```python
from build123d import *

# Parameters (mm, degrees)
SKETCH1_W           = 18.8
SKETCH1_H           = 14.8
BOSS_EXTRUDE1_DEPTH = 5.2
SKETCH2_W           = 1.2
SKETCH2_H           = 0.8
CUT_EXTRUDE1_DEPTH  = 19.287700785
SKETCH3_W           = 1.2
SKETCH3_H           = 0.8
CUT_EXTRUDE2_DEPTH  = 19.287700785
SKETCH4_W           = 1.2
SKETCH4_H           = 0.8
CUT_EXTRUDE3_DEPTH  = 19.287700785
SKETCH5_W           = 1.2
SKETCH5_H           = 0.8
CUT_EXTRUDE4_DEPTH  = 19.287700785
SKETCH6_W           = 1.2
SKETCH6_H           = 0.8
CUT_EXTRUDE5_DEPTH  = 19.287700785
SKETCH7_W           = 1.2
SKETCH7_H           = 0.8
CUT_EXTRUDE6_DEPTH  = 19.287700785
SKETCH8_W           = 1.2
SKETCH8_H           = 0.8
CUT_EXTRUDE7_DEPTH  = 19.287700785
SKETCH9_W           = 1.2
SKETCH9_H           = 0.8
CUT_EXTRUDE8_DEPTH  = 19.287700785
SKETCH10_W          = 1.2
SKETCH10_H          = 0.8
CUT_EXTRUDE9_DEPTH  = 19.287700785
RIB1_REACH          = 15.045
SKETCH11_WALL_W     = 29.289078174
SKETCH11_WALL_H     = 1
RIB2_REACH          = 15.045
SKETCH12_WALL_W     = 29.289078174
SKETCH12_WALL_H     = 1
RIB3_REACH          = 15.045
SKETCH13_WALL_W     = 29.289078174
SKETCH13_WALL_H     = 1
RIB4_REACH          = 15.045
SKETCH14_WALL_W     = 29.289078174
SKETCH14_WALL_H     = 1
RIB5_REACH          = 15.045
SKETCH15_WALL_W     = 29.289078174
SKETCH15_WALL_H     = 1
RIB6_REACH          = 15.045
SKETCH16_WALL_W     = 29.289078174
SKETCH16_WALL_H     = 1
RIB7_REACH          = 15.045
SKETCH17_WALL_W     = 29.289078174
SKETCH17_WALL_H     = 1
RIB8_REACH          = 15.045
SKETCH18_WALL_W     = 29.289078174
SKETCH18_WALL_H     = 1
RIB9_REACH          = 15.045
SKETCH19_WALL_W     = 29.289078174
SKETCH19_WALL_H     = 1
FILLET1_R           = 1
CHAMFER1_SIZE       = 0.5
FILLET2_START       = -8
FILLET2_DEPTH       = 16


with BuildPart() as part:
    # Sketch1 → Boss-Extrude1 (new body)
    with BuildSketch(Plane.XZ):
        Rectangle(SKETCH1_W, SKETCH1_H)
    extrude(amount=-BOSS_EXTRUDE1_DEPTH)

    # Sketch2 → Cut-Extrude1 (cut, through all)
    with BuildSketch(Plane(origin=(0, 0, -7.4), x_dir=(-1, 0, 0), z_dir=(0, 0, -1))):
        with Locations((-8, 4.8)):
            Rectangle(SKETCH2_W, SKETCH2_H)
    extrude(amount=-CUT_EXTRUDE1_DEPTH, mode=Mode.SUBTRACT)

    # Sketch3 → Cut-Extrude2 (cut, through all)
    with BuildSketch(Plane(origin=(0, 0, -7.4), x_dir=(-1, 0, 0), z_dir=(0, 0, -1))):
        with Locations((-6, 4.8)):
            Rectangle(SKETCH3_W, SKETCH3_H)
    extrude(amount=-CUT_EXTRUDE2_DEPTH, mode=Mode.SUBTRACT)

    # Sketch4 → Cut-Extrude3 (cut, through all)
    with BuildSketch(Plane(origin=(0, 0, -7.4), x_dir=(-1, 0, 0), z_dir=(0, 0, -1))):
        with Locations((-4, 4.8)):
            Rectangle(SKETCH4_W, SKETCH4_H)
    extrude(amount=-CUT_EXTRUDE3_DEPTH, mode=Mode.SUBTRACT)

    # Sketch5 → Cut-Extrude4 (cut, through all)
    with BuildSketch(Plane(origin=(0, 0, -7.4), x_dir=(-1, 0, 0), z_dir=(0, 0, -1))):
        with Locations((-2, 4.8)):
            Rectangle(SKETCH5_W, SKETCH5_H)
    extrude(amount=-CUT_EXTRUDE4_DEPTH, mode=Mode.SUBTRACT)

    # Sketch6 → Cut-Extrude5 (cut, through all)
    with BuildSketch(Plane(origin=(0, 0, -7.4), x_dir=(-1, 0, 0), z_dir=(0, 0, -1))):
        with Locations((0, 4.8)):
            Rectangle(SKETCH6_W, SKETCH6_H)
    extrude(amount=-CUT_EXTRUDE5_DEPTH, mode=Mode.SUBTRACT)

    # Sketch7 → Cut-Extrude6 (cut, through all)
    with BuildSketch(Plane(origin=(0, 0, -7.4), x_dir=(-1, 0, 0), z_dir=(0, 0, -1))):
        with Locations((2, 4.8)):
            Rectangle(SKETCH7_W, SKETCH7_H)
    extrude(amount=-CUT_EXTRUDE6_DEPTH, mode=Mode.SUBTRACT)

    # Sketch8 → Cut-Extrude7 (cut, through all)
    with BuildSketch(Plane(origin=(0, 0, -7.4), x_dir=(-1, 0, 0), z_dir=(0, 0, -1))):
        with Locations((4, 4.8)):
            Rectangle(SKETCH8_W, SKETCH8_H)
    extrude(amount=-CUT_EXTRUDE7_DEPTH, mode=Mode.SUBTRACT)

    # Sketch9 → Cut-Extrude8 (cut, through all)
    with BuildSketch(Plane(origin=(0, 0, -7.4), x_dir=(-1, 0, 0), z_dir=(0, 0, -1))):
        with Locations((6, 4.8)):
            Rectangle(SKETCH9_W, SKETCH9_H)
    extrude(amount=-CUT_EXTRUDE8_DEPTH, mode=Mode.SUBTRACT)

    # Sketch10 → Cut-Extrude9 (cut, through all)
    with BuildSketch(Plane(origin=(0, 0, -7.4), x_dir=(-1, 0, 0), z_dir=(0, 0, -1))):
        with Locations((8, 4.8)):
            Rectangle(SKETCH10_W, SKETCH10_H)
    extrude(amount=-CUT_EXTRUDE9_DEPTH, mode=Mode.SUBTRACT)

    # Sketch11 wall → Rib1 (add, up to next)
    with BuildSketch(Plane(origin=(4, 5, 0), x_dir=(1, 0, 0), z_dir=(0, -1, 0)), mode=Mode.PRIVATE) as rib1_sk1:
        Rectangle(SKETCH11_WALL_W, SKETCH11_WALL_H)
    rib1_tool1 = extrude(rib1_sk1.sketch, amount=RIB1_REACH, mode=Mode.PRIVATE) - part.part
    add(rib1_tool1.solids().sort_by_distance((4, 5, 0))[0])

    # Sketch12 wall → Rib2 (add, up to next)
    with BuildSketch(Plane(origin=(-4, 5, 0), x_dir=(1, 0, 0), z_dir=(0, -1, 0)), mode=Mode.PRIVATE) as rib2_sk1:
        Rectangle(SKETCH12_WALL_W, SKETCH12_WALL_H)
    rib2_tool1 = extrude(rib2_sk1.sketch, amount=RIB2_REACH, mode=Mode.PRIVATE) - part.part
    add(rib2_tool1.solids().sort_by_distance((-4, 5, 0))[0])

    # Sketch13 wall → Rib3 (add, up to next)
    with BuildSketch(Plane(origin=(-8, 5, 0), x_dir=(1, 0, 0), z_dir=(0, -1, 0)), mode=Mode.PRIVATE) as rib3_sk1:
        Rectangle(SKETCH13_WALL_W, SKETCH13_WALL_H)
    rib3_tool1 = extrude(rib3_sk1.sketch, amount=RIB3_REACH, mode=Mode.PRIVATE) - part.part
    add(rib3_tool1.solids().sort_by_distance((-8, 5, 0))[0])

    # Sketch14 wall → Rib4 (add, up to next)
    with BuildSketch(Plane(origin=(8, 5, 0), x_dir=(1, 0, 0), z_dir=(0, -1, 0)), mode=Mode.PRIVATE) as rib4_sk1:
        Rectangle(SKETCH14_WALL_W, SKETCH14_WALL_H)
    rib4_tool1 = extrude(rib4_sk1.sketch, amount=RIB4_REACH, mode=Mode.PRIVATE) - part.part
    add(rib4_tool1.solids().sort_by_distance((8, 5, 0))[0])

    # Sketch15 wall → Rib5 (add, up to next)
    with BuildSketch(Plane(origin=(2, 5, 0), x_dir=(1, 0, 0), z_dir=(0, -1, 0)), mode=Mode.PRIVATE) as rib5_sk1:
        Rectangle(SKETCH15_WALL_W, SKETCH15_WALL_H)
    rib5_tool1 = extrude(rib5_sk1.sketch, amount=RIB5_REACH, mode=Mode.PRIVATE) - part.part
    add(rib5_tool1.solids().sort_by_distance((2, 5, 0))[0])

    # Sketch16 wall → Rib6 (add, up to next)
    with BuildSketch(Plane(origin=(-2, 5, 0), x_dir=(1, 0, 0), z_dir=(0, -1, 0)), mode=Mode.PRIVATE) as rib6_sk1:
        Rectangle(SKETCH16_WALL_W, SKETCH16_WALL_H)
    rib6_tool1 = extrude(rib6_sk1.sketch, amount=RIB6_REACH, mode=Mode.PRIVATE) - part.part
    add(rib6_tool1.solids().sort_by_distance((-2, 5, 0))[0])

    # Sketch17 wall → Rib7 (add, up to next)
    with BuildSketch(Plane(origin=(6, 5, 0), x_dir=(1, 0, 0), z_dir=(0, -1, 0)), mode=Mode.PRIVATE) as rib7_sk1:
        Rectangle(SKETCH17_WALL_W, SKETCH17_WALL_H)
    rib7_tool1 = extrude(rib7_sk1.sketch, amount=RIB7_REACH, mode=Mode.PRIVATE) - part.part
    add(rib7_tool1.solids().sort_by_distance((6, 5, 0))[0])

    # Sketch18 wall → Rib8 (add, up to next)
    with BuildSketch(Plane.XZ.offset(-5), mode=Mode.PRIVATE) as rib8_sk1:
        Rectangle(SKETCH18_WALL_W, SKETCH18_WALL_H)
    rib8_tool1 = extrude(rib8_sk1.sketch, amount=RIB8_REACH, mode=Mode.PRIVATE) - part.part
    add(rib8_tool1.solids().sort_by_distance((0, 5, 0))[0])

    # Sketch19 wall → Rib9 (add, up to next)
    with BuildSketch(Plane(origin=(-6, 5, 0), x_dir=(1, 0, 0), z_dir=(0, -1, 0)), mode=Mode.PRIVATE) as rib9_sk1:
        Rectangle(SKETCH19_WALL_W, SKETCH19_WALL_H)
    rib9_tool1 = extrude(rib9_sk1.sketch, amount=RIB9_REACH, mode=Mode.PRIVATE) - part.part
    add(rib9_tool1.solids().sort_by_distance((-6, 5, 0))[0])

    # Fillet1
    fillet1_edges = [part.edges().sort_by_distance(p)[0] for p in [
        (9.4, 0, 0),
        (-9.4, 0, 0),
    ]]
    fillet(fillet1_edges, radius=FILLET1_R)

    # Chamfer1
    chamfer1_edges = [part.edges().sort_by_distance(p)[0] for p in [
        (-9.4, 3.1, 7.4),
        (9.4, 3.1, 7.4),
        (9.4, 3.1, -7.4),
        (-9.4, 3.1, -7.4),
        (0, 0, -7.4),
        (0, 0, 7.4),
        (-9.107106781, 0.292893219, 7.4),
        (9.107106781, 0.292893219, 7.4),
        (-9.107106781, 0.292893219, -7.4),
        (9.107106781, 0.292893219, -7.4),
    ]]
    chamfer(chamfer1_edges, length=CHAMFER1_SIZE)

    # Fillet2: read off the stored shape, not the designer's step
    # Fillet2 outline → Fillet2 (cut)
    with BuildSketch(Plane.XY.offset(FILLET2_START)):
        with BuildLine():
            Line((7.4, 5.2), (7.2, 5.2))
            ThreePointArc((7.2, 5.2), (7.341421356, 5.141421356), (7.4, 5))
            Line((7.4, 5), (7.4, 5.2))
        make_face()
        with BuildLine():
            ThreePointArc((6.6, 5), (6.658578644, 5.141421356), (6.8, 5.2))
            Line((6.8, 5.2), (6.6, 5.2))
            Line((6.6, 5.2), (6.6, 5))
        make_face()
        with BuildLine():
            Line((3.4, 5.2), (3.2, 5.2))
            ThreePointArc((3.2, 5.2), (3.341421356, 5.141421356), (3.4, 5))
            Line((3.4, 5), (3.4, 5.2))
        make_face()
        with BuildLine():
            ThreePointArc((2.6, 5), (2.658578644, 5.141421356), (2.8, 5.2))
            Line((2.8, 5.2), (2.6, 5.2))
            Line((2.6, 5.2), (2.6, 5))
        make_face()
        with BuildLine():
            Line((1.4, 5.2), (1.2, 5.2))
            ThreePointArc((1.2, 5.2), (1.341421356, 5.141421356), (1.4, 5))
            Line((1.4, 5), (1.4, 5.2))
        make_face()
        with BuildLine():
            ThreePointArc((0.6, 5), (0.658578644, 5.141421356), (0.8, 5.2))
            Line((0.8, 5.2), (0.6, 5.2))
            Line((0.6, 5.2), (0.6, 5))
        make_face()
        with BuildLine():
            Line((-7.4, 5.2), (-7.4, 5))
            ThreePointArc((-7.4, 5), (-7.341421356, 5.141421356), (-7.2, 5.2))
            Line((-7.2, 5.2), (-7.4, 5.2))
        make_face()
        with BuildLine():
            Line((-6.6, 5.2), (-6.8, 5.2))
            ThreePointArc((-6.8, 5.2), (-6.658578644, 5.141421356), (-6.6, 5))
            Line((-6.6, 5), (-6.6, 5.2))
        make_face()
        with BuildLine():
            Line((5.4, 5.2), (5.2, 5.2))
            ThreePointArc((5.2, 5.2), (5.341421356, 5.141421356), (5.4, 5))
            Line((5.4, 5), (5.4, 5.2))
        make_face()
        with BuildLine():
            ThreePointArc((4.6, 5), (4.658578644, 5.141421356), (4.8, 5.2))
            Line((4.8, 5.2), (4.6, 5.2))
            Line((4.6, 5.2), (4.6, 5))
        make_face()
        with BuildLine():
            Line((-8.6, 5.2), (-8.8, 5.2))
            ThreePointArc((-8.8, 5.2), (-8.658578644, 5.141421356), (-8.6, 5))
            Line((-8.6, 5), (-8.6, 5.2))
        make_face()
        with BuildLine():
            ThreePointArc((-9.4, 5), (-9.341421356, 5.141421356), (-9.2, 5.2))
            Line((-9.2, 5.2), (-9.4, 5.2))
            Line((-9.4, 5.2), (-9.4, 5))
        make_face()
        with BuildLine():
            Line((-5.4, 5.2), (-5.4, 5))
            ThreePointArc((-5.4, 5), (-5.341421356, 5.141421356), (-5.2, 5.2))
            Line((-5.2, 5.2), (-5.4, 5.2))
        make_face()
        with BuildLine():
            Line((-4.6, 5.2), (-4.8, 5.2))
            ThreePointArc((-4.8, 5.2), (-4.658578644, 5.141421356), (-4.6, 5))
            Line((-4.6, 5), (-4.6, 5.2))
        make_face()
        with BuildLine():
            Line((-3.4, 5.2), (-3.4, 5))
            ThreePointArc((-3.4, 5), (-3.341421356, 5.141421356), (-3.2, 5.2))
            Line((-3.2, 5.2), (-3.4, 5.2))
        make_face()
        with BuildLine():
            Line((-2.6, 5.2), (-2.8, 5.2))
            ThreePointArc((-2.8, 5.2), (-2.658578644, 5.141421356), (-2.6, 5))
            Line((-2.6, 5), (-2.6, 5.2))
        make_face()
        with BuildLine():
            Line((-1.4, 5.2), (-1.4, 5))
            ThreePointArc((-1.4, 5), (-1.341421356, 5.141421356), (-1.2, 5.2))
            Line((-1.2, 5.2), (-1.4, 5.2))
        make_face()
        with BuildLine():
            Line((-0.6, 5.2), (-0.8, 5.2))
            ThreePointArc((-0.8, 5.2), (-0.658578644, 5.141421356), (-0.6, 5))
            Line((-0.6, 5), (-0.6, 5.2))
        make_face()
        with BuildLine():
            Line((8.6, 5.2), (8.6, 5))
            ThreePointArc((8.6, 5), (8.658578644, 5.141421356), (8.8, 5.2))
            Line((8.8, 5.2), (8.6, 5.2))
        make_face()
        with BuildLine():
            Line((9.4, 5.2), (9.2, 5.2))
            ThreePointArc((9.2, 5.2), (9.341421356, 5.141421356), (9.4, 5))
            Line((9.4, 5), (9.4, 5.2))
        make_face()
    extrude(amount=FILLET2_DEPTH, mode=Mode.SUBTRACT)


solid = part.part
```
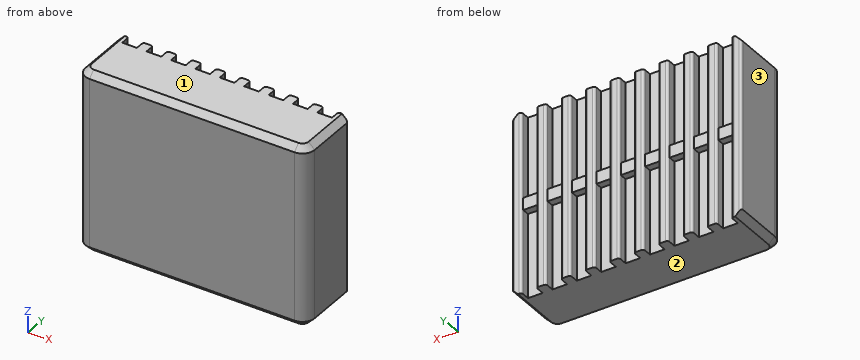
Verification items for the finished model (mm, model axes). Face numbers are marked on the shaded views. Round coordinates to 2 decimals unless told otherwise and drop trailing zeros. Loops run counter-clockwise (first coordinate to the right, second up) from the corner with the lowest first, then second, coordinate; pieces in that order, holes last. Notation, with made-up numbers: (-40, 19) -> (-22, 19) arc R29 ccw to (-22, 48) -> close; hole circle Ø7 at (24, 73.5). An arc over 180 degrees is marked (long way). Answer as a JSON object with one key per item and string values.
Q1. Scan lines: line 1 (Y direction, x = 6.5, z = -6.25); line 2 (Z direction, x = -0.25, y = 4.6); line 3 (Y direction, x = -4.75, z = -5). Record each from-to range of solid material in increasing order. Write a range as from..to.
Data:
{"line 1": "y = 0..4.4", "line 2": "z = -0.5..0.5", "line 3": "y = 0..5.19"}
Q2. Section check A-A (x = 6.25). Record the boundary of the cut face in (y, z), then the cut area to 3 significant figures.
Data:
{"outline": "(0, -6.9) -> (0.5, -7.4) -> (4.4, -7.4) -> (4.4, -0.5) -> (5, -0.5) -> (5, 0.5) -> (4.4, 0.5) -> (4.4, 7.4) -> (0.5, 7.4) -> (0, 6.9) -> close", "area": "65.5 mm2"}
Q3. Go/stop test with flat-tipped pins: P1, Ø0.6, axis at x = 8, z = 3.5, coming from the +Y side; P2, Ø0.7, axis at x = -6, y = 5, coming from the -Z side; P3, Ø1.3, axis at x = -1.5, z = -4, coming from the +Y side. Record where each tip stops, or that it passes through.
Data:
{"P1": "stops at y = 4.4", "P2": "stops at z = -0.5", "P3": "stops at y = 5.2"}
Q4. Draft check along Z on the marked faces 1, 2 and 3. Enter one of: pulls with the +Z half, pulls with the -Z half, needs draft (parallel to the pull), parting line crosses it, or undercut.
Data:
{"face 1": "pulls with the +Z half", "face 2": "pulls with the -Z half", "face 3": "needs draft"}
